Could you check a few things on this model? Use its own coordinates, in mm. A direction names the side the tool comes from. Round coordinates to 2 decimals unless told otherwise and drop trailing zeros. Loops run counter-clockwise (first coordinate to the right, second up) from the corner with the lowest first, then second, coordinate; pieces in that order, holes last. Notation, with made-up numbers: (-13, 0.25) - (6, 0.25) arc R27 ccw to (6, 31.25) - close; hole circle Ø9 at (-28.5, -36). An arc over 180 degrees is marked (long way). Put each result on its own line as item: value. Start each with the question number.
Autodesk Inventor part; units mm, degrees
ref_plane "YZ Plane" through (0, 0, 0) normal (1, 0, 0) x (0, 1, 0)
ref_plane "XZ Plane" through (0, 0, 0) normal (0, 1, 0) x (-1, 0, 0)
ref_plane "XY Plane" through (0, 0, 0) normal (0, 0, 1) x (1, 0, 0)
sketch "Szkic1" plane through (0, 0, 0) normal (0, 1, 0) x (-1, 0, 0)
  line L0 (-75, 75) -> (75, 75)
  line L1 (75, 75) -> (75, -75)
  line L2 (75, -75) -> (-75, -75)
  line L3 (-75, -75) -> (-75, 75)
  line L4 (-75, 75) -> (75, -75) construction
  line L5 (75, 75) -> (-75, -75) construction
  point P0 (0, 0)
  dimension "d0" = 150
  dimension "d1" = 150
extrude "Wyciągnięcie proste1" add sketch "Szkic1" along normal blind 5
sketch "Szkic2" plane through (75, 0, 75) normal (1, 0, 0) x (0, 0, -1)
  line L0 (0, 5) -> (150, 5)
  line L1 (150, 5) -> (150, 55)
  line L2 (150, 55) -> (0, 55)
  line L3 (0, 55) -> (0, 5)
  line L4 (50, 55) -> (100, 55)
  point P0 (75, 0)
  dimension "d4" = 50
extrude "Wyciągnięcie proste2" add sketch "Szkic2" against normal blind 5
sketch "Szkic3" plane through (-75, 0, -75) normal (-1, 0, 0) x (0, 0, 1)
  line L0 (0, 5) -> (150, 5)
  line L1 (150, 5) -> (150, 55)
  line L2 (150, 55) -> (0, 55)
  line L3 (0, 55) -> (0, 5)
  point P0 (75, 0)
  dimension "d7" = 50
extrude "Wyciągnięcie proste3" add sketch "Szkic3" against normal blind 5
sketch "Szkic4" plane through (-75, 0, 75) normal (0, 0, 1) x (1, 0, 0)
  line L0 (5, 5) -> (145, 5)
  line L1 (145, 5) -> (145, 55)
  line L2 (145, 55) -> (5, 55)
  line L3 (5, 55) -> (5, 5)
  point P0 (75, 0)
extrude "Wyciągnięcie proste4" add sketch "Szkic4" against normal blind 5
sketch "Szkic5" plane through (75, 0, -75) normal (0, 0, -1) x (-1, 0, 0)
  line L0 (5, 5) -> (145, 5)
  line L1 (145, 5) -> (145, 55)
  line L2 (145, 55) -> (5, 55)
  line L3 (5, 55) -> (5, 5)
  point P0 (75, 0)
extrude "Wyciągnięcie proste5" add sketch "Szkic5" against normal blind 5
sketch "Szkic10" plane through (-75, 0, 75) normal (0, 0, 1) x (1, 0, 0)
  circle A0 centre (30, 28) radius 1.5
  circle A1 centre (120, 28) radius 1.5
  point P0 (75, 0)
  dimension "d53" = 3
  dimension "d54" = 3
hole "Otwór5" at (45, 28, 75) at (-45, 28, 75) direction (0, 0, -1) diameter 3 depth 8 tip angle 118
sketch "Szkic11" plane through (75, 0, -75) normal (0, 0, -1) x (-1, 0, 0)
  circle A0 centre (30, 28) radius 1.5
  circle A1 centre (120, 28) radius 1.5
  point P0 (75, 0)
  dimension "d62" = 3
  dimension "d63" = 3
hole "Otwór6" at (45, 28, -75) at (-45, 28, -75) direction (0, 0, 1) diameter 3 depth 8 tip angle 118
sketch "Szkic12" plane through (70, 0, 75) normal (-1, 0, 0) x (0, 0, 1)
  line L0 (-145, 55) -> (-145, 5)
  line L1 (-5, 5) -> (-145, 5)
  line L2 (-5, 5) -> (-5, 55)
  line L3 (-5, 55) -> (-145, 55)
  point P0 (-75, 0)
sketch "Szkic13" plane through (75, 0, 75) normal (1, 0, 0) x (0, 0, -1)
  line L0 (150, 0) -> (0, 0)
  line L1 (150, 0) -> (150, 55)
  line L2 (150, 55) -> (0, 55)
  line L3 (0, 0) -> (0, 55)
  point P0 (75, 0)
sketch "Szkic14" plane through (75, 0, 75) normal (1, 0, 0) x (0, 0, -1)
  line L0 (150, 55) -> (0, 55)
  line L1 (55, 55) -> (95, 55)
  line L2 (95, 55) -> (95, 39)
  line L3 (95, 39) -> (55, 39)
  line L4 (55, 39) -> (55, 55)
  point P0 (75, 0)
  dimension "d73" = 40
  dimension "d74" = 16
extrude "Wyciągnięcie proste6" cut sketch "Szkic14" against normal blind 5
sketch "Szkic15" plane through (75, 0, -75) normal (0, 0, -1) x (-1, 0, 0)
  line L0 (150, 55) -> (0, 55)
  line L1 (55, 55) -> (95, 55)
  line L2 (95, 55) -> (95, 39)
  line L3 (95, 39) -> (55, 39)
  line L4 (55, 39) -> (55, 55)
  point P0 (75, 0)
  dimension "d77" = 40
  dimension "d78" = 16
extrude "Wyciągnięcie proste7" cut sketch "Szkic15" against normal blind 5
sketch "Szkic16" plane through (-75, 0, 75) normal (0, 0, 1) x (1, 0, 0)
  line L0 (150, 55) -> (0, 55)
  line L1 (55, 55) -> (95, 55)
  line L2 (95, 55) -> (95, 39)
  line L3 (95, 39) -> (55, 39)
  line L4 (55, 39) -> (55, 55)
  point P0 (75, 0)
  dimension "d81" = 40
  dimension "d82" = 16
extrude "Wyciągnięcie proste8" cut sketch "Szkic16" against normal blind 5
sketch "Szkic17" plane through (-75, 0, -75) normal (-1, 0, 0) x (0, 0, 1)
  line L0 (150, 55) -> (0, 55)
  line L1 (55, 55) -> (95, 55)
  line L2 (95, 55) -> (95, 39)
  line L3 (95, 39) -> (55, 39)
  line L4 (55, 39) -> (55, 55)
  point P0 (75, 0)
  dimension "d85" = 40
  dimension "d86" = 16
extrude "Wyciągnięcie proste9" cut sketch "Szkic17" against normal blind 5
properties part number "korpus" material "Stal"
Item 1: Suppose I cut it at A-A, the plane y = 24. List the corners of the cut face in (x, z) for me.
Item 2: Suppose I cut it at B-B, the plane z = -13. List the corners of the cut face in (x, y) for me, then the cut area to 3 significant figures.
Item 3: Suppose I cut it at C-C, the plane x = 12. List the corners of the cut face in (y, z) for me.
Item 4: Will these pins go through, and if not, where does the flat tip stop? P1, Ø4, axis at x = -71.5, z = -0.5, coming from the +Y side; P2, Ø12, axis at x = -57.5, z = 37.5, coming from the -Y side.
Item 5: On a 3-axis mill with a long thin cutter (end or side, diameter ignored), from which of +Z, -Z, +X, -X, +Y, -Y can I reach the whole of each face in a straight line? I mean faces 3 (the face through (1, 28, -75)), 4 (the face through (73, 39, 0)), 5 (the face through (20, 47, 73)), 6 (the face through (-70, 30, -1)), 7 (the face through (-72, 55, 58)). Say none if no direction works.
Item 6: Thinking about a two-plate mould opening in X: for faces 1 (the face through (1, 0, 1)), 2 (the face through (-20, 47, 73)), which applies, released by +X, released by -X, zero draft, split by the parting line, or undercut?
Item 7: Suppose I cut it at D-D, the plane y = 50.5. List the corners of the cut face in (x, z) for me, then the cut area to 3 significant figures.
Item 8: I need wall thicknesses on line 1 (X direction, y = 28, z = 72.3); line 2 (X direction, y = 6, z = 68). Which ranges of each line are inside material? Lowest first, please. Write a range as from..to.
Numbers:
1. outline: (-75, -75) - (75, -75) - (75, 75) - (-75, 75) - close; hole (-70, -70) - (70, -70) - (70, 70) - (-70, 70) - close
2. outline: (-75, 0) - (75, 0) - (75, 39) - (70, 39) - (70, 5) - (-70, 5) - (-70, 39) - (-75, 39) - close
2. area: 1,090 mm^2
3. outline: (0, -75) - (39, -75) - (39, -70) - (5, -70) - (5, 70) - (39, 70) - (39, 75) - (0, 75) - close
4. P1: y = 39
4. P2: y = 0
5. face 3: -Z, +X, -X, +Y, -Y
5. face 4: +X, -X, +Y
5. face 5: +Z, -Z, +Y
5. face 6: +Y
5. face 7: +Z, -Z, +X, -X, +Y
6. face 1: zero draft
6. face 2: undercut
7. outline: (-75, -75) - (-20, -75) - (-20, -70) - (-70, -70) - (-70, -20) - (-75, -20) - close; (-75, 20) - (-70, 20) - (-70, 70) - (-20, 70) - (-20, 75) - (-75, 75) - close; (20, -75) - (75, -75) - (75, -20) - (70, -20) - (70, -70) - (20, -70) - close; (20, 70) - (70, 70) - (70, 20) - (75, 20) - (75, 75) - (20, 75) - close
7. area: 2,100 mm^2
8. line 1: -75..-46.5, -43.5..43.5, 46.5..75
8. line 2: -75..-70, 70..75
